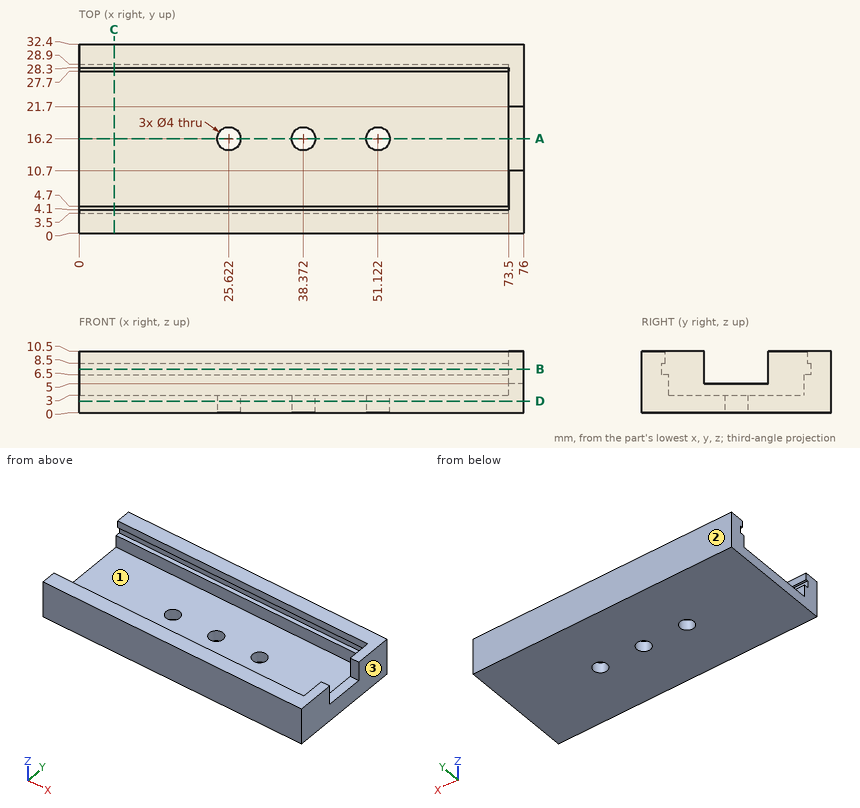
Drawing for the job (mm, zero at the part's lowest x, y, z). Round coordinates to 2 decimals unless told otherwise and drop trailing zeros. Loops run counter-clockwise (first coordinate to the right, second up) from the corner with the lowest first, then second, coordinate; pieces in that order, holes last. Notation, with made-up numbers: (-26, -19) -> (-9, -19) arc R25 cw to (-9, 6) -> close; hole circle Ø1 at (50, -13). An arc over 180 degrees is marked (long way). Answer as CSV lines item,"result". Start each with the question number.
1) Mould opens along Y. For the marked faces 1, 2 and 3 say: +Y half, -Y half, draft (parallel to the pull), parting line (faces both ways), or undercut.
2) Slice it at C-C (x = 6). List the corners of the cut face in (y, z), plus the area to 4 significant figures.
3) Slice it at A-A (y = 16.2). List the corners of the cut face in (x, z).
4) Probe line 1 along X through (y, z) = (16.2, 1.45); line 2 along Y through (x, z) = (24.5, 4); line 3 along Y through (x, z) = (35, 8.75). List the from-to ranges inside material, lowest first.
5) Slice it at B-B (z = 7.5). List the corners of the cut face in (x, y), plus the area to 3 significant figures.
6) Slice it at D-D (z = 2). List the corners of the cut face in (x, y), plus the area to 3 significant figures.
7) Pin check, flat tips, straight feed: P1, Ø6.5, axis at x = 25.622, y = 16.2, coming from the +Z side; P2, Ø0.8, axis at x = 75, y = 14, coming from the +Z side. Stop position of each tip, or through.
Filled in:
1,face 1,"undercut"
1,face 2,"+Y half"
1,face 3,"draft"
2,outline,"(0, 0) -> (32.4, 0) -> (32.4, 10.5) -> (28.3, 10.5) -> (28.3, 8.5) -> (28.9, 8.5) -> (28.9, 6.5) -> (27.7, 6.5) -> (27.7, 3) -> (4.7, 3) -> (4.7, 6.5) -> (3.5, 6.5) -> (3.5, 8.5) -> (4.1, 8.5) -> (4.1, 10.5) -> (0, 10.5) -> close"
2,area,"160.5 mm2"
3,outline,"(0, 0) -> (23.62, 0) -> (23.62, 3) -> (0, 3) -> close; (27.62, 0) -> (36.37, 0) -> (36.37, 3) -> (27.62, 3) -> close; (40.37, 0) -> (49.12, 0) -> (49.12, 3) -> (40.37, 3) -> close; (53.12, 0) -> (76, 0) -> (76, 5) -> (73.5, 5) -> (73.5, 3) -> (53.12, 3) -> close"
4,line 1,"x = 0 to 23.62, 27.62 to 36.37, 40.37 to 49.12, 53.12 to 76"
4,line 2,"y = 0 to 4.7, 27.7 to 32.4"
4,line 3,"y = 0 to 4.1, 28.3 to 32.4"
5,outline,"(0, 0) -> (76, 0) -> (76, 10.7) -> (73.5, 10.7) -> (73.5, 3.5) -> (0, 3.5) -> close; (0, 28.9) -> (73.5, 28.9) -> (73.5, 21.7) -> (76, 21.7) -> (76, 32.4) -> (0, 32.4) -> close"
5,area,"568 mm2"
6,outline,"(0, 0) -> (76, 0) -> (76, 32.4) -> (0, 32.4) -> close; hole circle Ø4 at (25.62, 16.2); hole circle Ø4 at (38.37, 16.2); hole circle Ø4 at (51.12, 16.2)"
6,area,"2,420 mm2"
7,P1,"stops at z = 3"
7,P2,"stops at z = 5"
